```python
from build123d import *

# Parameters (mm, degrees)
SKETCH2_R           = 13.25
SKETCH2_R_2         = 12.25
BOSS_EXTRUDE1_DEPTH = 50
SKETCH4_W           = 5
SKETCH4_H           = 45
CUT_EXTRUDE2_DEPTH  = 5
SKETCH6_R           = 17
SKETCH6_R_2         = 8
BOSS_EXTRUDE3_DEPTH = 2.5
BOSS_EXTRUDE4_DEPTH = 5
SCALE1_SCALE        = 0.8


with BuildPart() as part:
    # Sketch2 → Boss-Extrude1 (new body)
    with BuildSketch(Plane(origin=(0, 0, 0), x_dir=(1, 0, 0), z_dir=(0, 1, 0))):
        with Locations(Location((0, 0, 0), (0, 0, 270))):
            Circle(SKETCH2_R)
        with Locations(Location((0, 0, 0), (0, 0, 270))):
            Circle(SKETCH2_R_2, mode=Mode.SUBTRACT)
    extrude(amount=BOSS_EXTRUDE1_DEPTH)

    # Sketch4 → Cut-Extrude2 (cut)
    with BuildSketch(Plane(origin=(13.25, 0, 0), x_dir=(0, 0, -1), z_dir=(1, 0, 0))):
        with BuildLine():
            ThreePointArc((-3, 45), (-3.732233047, 46.767766953), (-5.5, 47.5))
            Line((-5.5, 47.5), (-5.5, 42.5))
            ThreePointArc((-5.5, 42.5), (-3.732233047, 43.232233047), (-3, 45))
        make_face()
        with BuildLine():
            Line((-5.5, 42.5), (-5.5, 47.5))
            ThreePointArc((-5.5, 47.5), (-8, 45), (-5.5, 42.5))
        make_face()
        with Locations((0, 25)):
            Rectangle(SKETCH4_W, SKETCH4_H)
        with BuildLine():
            ThreePointArc((8, 5), (7.267766953, 6.767766953), (5.5, 7.5))
            Line((5.5, 7.5), (5.5, 2.5))
            ThreePointArc((5.5, 2.5), (7.267766953, 3.232233047), (8, 5))
        make_face()
        with BuildLine():
            Line((5.5, 2.5), (5.5, 7.5))
            ThreePointArc((5.5, 7.5), (3, 5), (5.5, 2.5))
        make_face()
        with BuildLine():
            Line((5.5, 7.5), (2.5, 7.5))
            Line((2.5, 7.5), (2.5, 2.5))
            Line((2.5, 2.5), (5.5, 2.5))
            ThreePointArc((5.5, 2.5), (3, 5), (5.5, 7.5))
        make_face()
        with BuildLine():
            Line((-2.5, 42.5), (-2.5, 47.5))
            Line((-2.5, 47.5), (-5.5, 47.5))
            ThreePointArc((-5.5, 47.5), (-3.732233047, 46.767766953), (-3, 45))
            ThreePointArc((-3, 45), (-3.732233047, 43.232233047), (-5.5, 42.5))
            Line((-5.5, 42.5), (-2.5, 42.5))
        make_face()
    extrude(amount=-CUT_EXTRUDE2_DEPTH, mode=Mode.SUBTRACT)

    # Sketch6 → Boss-Extrude3 (add)
    with BuildSketch(Plane(origin=(0, 50, 0), x_dir=(1, 0, 0), z_dir=(0, 1, 0))):
        with Locations(Location((0, 0, 0), (0, 0, 270))):
            Circle(SKETCH6_R)
        with Locations(Location((0, 0, 0), (0, 0, 270))):
            Circle(SKETCH6_R_2, mode=Mode.SUBTRACT)
    extrude(amount=BOSS_EXTRUDE3_DEPTH)

    # Sketch7 → Boss-Extrude4 (add)
    with BuildSketch(Plane(origin=(0, 52.5, 0), x_dir=(1, 0, 0), z_dir=(0, 1, 0))):
        with BuildLine():
            ThreePointArc((9.369164851, -9.369164851), (8.037023703, -10.534170589), (6.561511052, -11.51125852))
            Line((6.561511052, -11.51125852), (8.329278005, -13.279025473))
            Line((8.329278005, -13.279025473), (13.279025473, -8.329278005))
            Line((13.279025473, -8.329278005), (11.51125852, -6.561511052))
            ThreePointArc((11.51125852, -6.561511052), (10.534170589, -8.037023703), (9.369164851, -9.369164851))
        make_face()
        with BuildLine():
            ThreePointArc((-6.561511052, -11.51125852), (-8.037023703, -10.534170589), (-9.369164851, -9.369164851))
            ThreePointArc((-9.369164851, -9.369164851), (-10.534170589, -8.037023703), (-11.51125852, -6.561511052))
            Line((-11.51125852, -6.561511052), (-13.279025473, -8.329278005))
            Line((-13.279025473, -8.329278005), (-8.329278005, -13.279025473))
            Line((-8.329278005, -13.279025473), (-6.561511052, -11.51125852))
        make_face()
        with BuildLine():
            Line((-13.279025473, 8.329278005), (-11.51125852, 6.561511052))
            ThreePointArc((-11.51125852, 6.561511052), (-10.534170589, 8.037023703), (-9.369164851, 9.369164851))
            ThreePointArc((-9.369164851, 9.369164851), (-8.037023703, 10.534170589), (-6.561511052, 11.51125852))
            Line((-6.561511052, 11.51125852), (-8.329278005, 13.279025473))
            Line((-8.329278005, 13.279025473), (-13.279025473, 8.329278005))
        make_face()
        with BuildLine():
            ThreePointArc((-6.561511052, 11.51125852), (-8.037023703, 10.534170589), (-9.369164851, 9.369164851))
            Line((-9.369164851, 9.369164851), (-5.168070815, 9.369164851))
            Line((-5.168070815, 9.369164851), (-4.793744099, 9.743491567))
            Line((-4.793744099, 9.743491567), (-6.561511052, 11.51125852))
        make_face()
        with BuildLine():
            Line((-9.743491567, 4.793744099), (-9.369164851, 5.168070815))
            Line((-9.369164851, 5.168070815), (-9.369164851, 9.369164851))
            ThreePointArc((-9.369164851, 9.369164851), (-10.534170589, 8.037023703), (-11.51125852, 6.561511052))
            Line((-11.51125852, 6.561511052), (-9.743491567, 4.793744099))
        make_face()
        Polygon((-9.369164851, 9.369164851), (-9.369164851, 5.168070815), (-5.168070815, 9.369164851), align=None)
        with BuildLine():
            Line((-5.168070815, -9.369164851), (-9.369164851, -9.369164851))
            ThreePointArc((-9.369164851, -9.369164851), (-8.037023703, -10.534170589), (-6.561511052, -11.51125852))
            Line((-6.561511052, -11.51125852), (-4.793744099, -9.743491567))
            Line((-4.793744099, -9.743491567), (-5.168070815, -9.369164851))
        make_face()
        Polygon((-9.369164851, -5.168070815), (-9.369164851, -9.369164851), (-5.168070815, -9.369164851), align=None)
        with BuildLine():
            ThreePointArc((-11.51125852, -6.561511052), (-10.534170589, -8.037023703), (-9.369164851, -9.369164851))
            Line((-9.369164851, -9.369164851), (-9.369164851, -5.168070815))
            Line((-9.369164851, -5.168070815), (-9.743491567, -4.793744099))
            Line((-9.743491567, -4.793744099), (-11.51125852, -6.561511052))
        make_face()
        with BuildLine():
            Line((9.369164851, -5.168070815), (9.369164851, -9.369164851))
            ThreePointArc((9.369164851, -9.369164851), (10.534170589, -8.037023703), (11.51125852, -6.561511052))
            Line((11.51125852, -6.561511052), (9.743491567, -4.793744099))
            Line((9.743491567, -4.793744099), (9.369164851, -5.168070815))
        make_face()
        Polygon((9.369164851, -5.168070815), (5.168070815, -9.369164851), (9.369164851, -9.369164851), align=None)
        with BuildLine():
            Line((9.369164851, -9.369164851), (5.168070815, -9.369164851))
            Line((5.168070815, -9.369164851), (4.793744099, -9.743491567))
            Line((4.793744099, -9.743491567), (6.561511052, -11.51125852))
            ThreePointArc((6.561511052, -11.51125852), (8.037023703, -10.534170589), (9.369164851, -9.369164851))
        make_face()
        with BuildLine():
            ThreePointArc((6.561511052, 11.51125852), (8.037023703, 10.534170589), (9.369164851, 9.369164851))
            ThreePointArc((9.369164851, 9.369164851), (10.534170589, 8.037023703), (11.51125852, 6.561511052))
            Line((11.51125852, 6.561511052), (13.279025473, 8.329278005))
            Line((13.279025473, 8.329278005), (8.329278005, 13.279025473))
            Line((8.329278005, 13.279025473), (6.561511052, 11.51125852))
        make_face()
        with BuildLine():
            Line((4.793744099, 9.743491567), (5.168070815, 9.369164851))
            Line((5.168070815, 9.369164851), (9.369164851, 9.369164851))
            ThreePointArc((9.369164851, 9.369164851), (8.037023703, 10.534170589), (6.561511052, 11.51125852))
            Line((6.561511052, 11.51125852), (4.793744099, 9.743491567))
        make_face()
        Polygon((5.168070815, 9.369164851), (9.369164851, 5.168070815), (9.369164851, 9.369164851), align=None)
        with BuildLine():
            Line((9.369164851, 9.369164851), (9.369164851, 5.168070815))
            Line((9.369164851, 5.168070815), (9.743491567, 4.793744099))
            Line((9.743491567, 4.793744099), (11.51125852, 6.561511052))
            ThreePointArc((11.51125852, 6.561511052), (10.534170589, 8.037023703), (9.369164851, 9.369164851))
        make_face()
    extrude(amount=BOSS_EXTRUDE4_DEPTH)


with BuildPart() as part_1:
    # Scale1: scaled about (-0.56553808, 35.88383974, 2.07e-07)
    add(part.part.scale(SCALE1_SCALE).moved(Location((-0.113107616, 7.176767948, 4.1e-08))))


solid = part_1.part
```
Work out the finished part from the listing and answer in its coordinate system (mm). A direction names the side the tool comes from. Coordinates: 2 decimals unless noted, no trailing zeros. Order: outer loops, then holes, each group sorted by start corner. A loop starts at its lowest first (then second) coordinate and runs counter-clockwise, first axis right, second up. Notation, with made-up numbers: (-29, 40.25) - (-22, 40.25) arc R31 cw to (-22, 64.25) - close; hole circle Ø4 at (-22, 5). An arc over 180 degrees is marked (long way). Answer as a JSON object with one key per item and string values.
1. Consider line 1 (X direction, y = 48.05, z = 0); line 2 (Y direction, x = -6, z = -5.5); line 3 (Y direction, x = -6.75, z = 10.25). Determine where each line is inside the solid, lowest interval first.
Output values:
{"line 1": "x = -13.71 to -6.51, 6.29 to 13.49", "line 2": "y = 47.18 to 49.18", "line 3": "y = 47.18 to 53.18"}
2. Each of these flat-tipped pins is pushed along its axis until it touches: P1, Ø5, axis at y = 39, z = 10.5, coming from the +X side; P2, Ø5, axis at x = 6.5, y = 31, coming from the -Z side; P3, Ø12, axis at y = 31.5, z = 5, coming from the -X side. Where does it stop, or does it pass through?
Output values:
{"P1": "stops at x = 6.84", "P2": "stops at z = -9.77", "P3": "stops at x = -10.71"}
3. Find section B-B on x = 4.25. Determine the outline of the cut face in (y, z).
Output values:
{"outline": "(7.18, -9.66) - (47.18, -9.66) - (47.18, -12.88) - (49.18, -12.88) - (49.18, -8.32) - (53.18, -8.32) - (53.18, -7.27) - (49.18, -7.27) - (49.18, -4.68) - (47.18, -4.68) - (47.18, -8.78) - (7.18, -8.78) - close; (7.18, 8.78) - (47.18, 8.78) - (47.18, 4.68) - (49.18, 4.68) - (49.18, 7.27) - (53.18, 7.27) - (53.18, 8.32) - (49.18, 8.32) - (49.18, 12.88) - (47.18, 12.88) - (47.18, 9.66) - (7.18, 9.66) - close"}
4. The mould has two halves that part along Y. Classify faces 5 (the face through (-9, 7.177, -5)), 6 (the face through (-5.322, 48.163, 12.563)), 7 (the face through (-3, 49.177, 6)), 8 (the face through (9.5, 13.177, -3.2)): +Y half, -Y half, draft (parallel to the pull), parting line (faces both ways), or undercut.
Output values:
{"face 5": "-Y half", "face 6": "draft", "face 7": "+Y half", "face 8": "undercut"}
5. Find section C-C on x = -5.75. Determine the outline of the cut face in (y, z).
Output values:
{"outline": "(7.18, -8.98) - (47.18, -8.98) - (47.18, -12.38) - (49.18, -12.38) - (49.18, -9.6) - (53.18, -9.6) - (53.18, -5.99) - (49.18, -5.99) - (49.18, -3.03) - (47.18, -3.03) - (47.18, -8.02) - (7.18, -8.02) - close; (7.18, 8.02) - (47.18, 8.02) - (47.18, 3.03) - (49.18, 3.03) - (49.18, 5.99) - (53.18, 5.99) - (53.18, 9.6) - (49.18, 9.6) - (49.18, 12.38) - (47.18, 12.38) - (47.18, 8.98) - (7.18, 8.98) - close"}
6. A tool of negligible diameter and unlimited length cuts with its end or side. For faces 1 (the face through (8.502, 51.149, 8.671)), 2 (the face through (-5.382, 51.149, 9.229)), 3 (the face through (-8.7, 51.1, -8.7)), 4 (the face through (-9.302, 51.149, 5.229)), from which of +Z, -Z, +X, -X, +Y, -Y can it reach the whole face along a straight path? Write none if from no direction.
Output values:
{"face 1": "+Z, +X, +Y", "face 2": "+Z, +Y", "face 3": "-Z, -X, +Y", "face 4": "-X, +Y"}
7. Find section A-A on z = 0. Determine the outline of the cut face in (x, y), plus the area to 3 significant figures.
Output values:
{"outline": "(-13.71, 47.18) - (-10.71, 47.18) - (-10.71, 7.18) - (-9.91, 7.18) - (-9.91, 47.18) - (-6.51, 47.18) - (-6.51, 49.18) - (-13.71, 49.18) - close; (6.29, 47.18) - (9.69, 47.18) - (9.69, 45.18) - (10.49, 45.18) - (10.49, 47.18) - (13.49, 47.18) - (13.49, 49.18) - (6.29, 49.18) - close; (9.69, 7.18) - (10.49, 7.18) - (10.49, 9.18) - (9.69, 9.18) - close", "area": "64.0 mm²"}
8. Find section D-D on y = 39.5. Determine the outline of the cut face in (x, z).
Output values:
{"outline": "(9.48, -2) arc R9.8 cw (long way) to (9.48, 2) - (10.3, 2) arc R10.6 ccw (long way) to (10.3, -2) - close"}
